```python
from build123d import *

# Parameters (mm, degrees)
SKETCH_1_R      = 16
SKETCH_1_R_2    = 4.5
SKETCH_1_R_3    = 1.85
EXTRUDE_1_DEPTH = 2


with BuildPart() as part:
    # 草图1 → 凸台-拉伸1 (new, symmetric)
    with BuildSketch(Plane.XY):
        Circle(SKETCH_1_R)
        Circle(SKETCH_1_R_2, mode=Mode.SUBTRACT)
        with Locations((-12, 0)):
            Circle(SKETCH_1_R_3, mode=Mode.SUBTRACT)
        with Locations((12, 0)):
            Circle(SKETCH_1_R_3, mode=Mode.SUBTRACT)
        with BuildLine():
            Line((-1, 6), (-1, 11))
            ThreePointArc((-1, 11), (0, 12), (1, 11))
            Line((1, 11), (1, 6))
            Line((1, 6), (-1, 6))
        make_face(mode=Mode.SUBTRACT)
        with BuildLine():
            Line((1, -6), (1, -11))
            ThreePointArc((1, -11), (0, -12), (-1, -11))
            Line((-1, -11), (-1, -6))
            Line((-1, -6), (1, -6))
        make_face(mode=Mode.SUBTRACT)
    extrude(amount=EXTRUDE_1_DEPTH, both=True)


solid = part.part
```
Read the model definition and answer for the solid it produces. Units are mm, in the model's axes. A direction names the side the tool comes from. Give positions to 0.01 mm unless a question says otherwise; leave off trailing zeros. Write each loop counter-clockwise with the first axis right and the second up, starting at its lowest first coordinate (ties: lowest second). Pieces come first, ordered by that corner, then holes. Notation, with made-up numbers: (-1, 12.5) -> (5, 12.5) arc R28 cw to (5, 45.5) -> close; hole circle Ø2 at (-7, -40). An arc over 180 degrees is marked (long way). Answer in a Markdown table with one row per item.
1) Section B-B on z = 0.8 is taken. Give the vertices of the cut face in (x, y).
Results list:
| item | result |
|---|---|
| outline | circle Ø32 at (0, 0); hole circle Ø3.7 at (-12, 0); hole circle Ø9 at (0, 0); hole (-1, -11) arc R1 ccw to (1, -11) -> (1, -6) -> (-1, -6) -> close; hole (-1, 6) -> (1, 6) -> (1, 11) arc R1 ccw to (-1, 11) -> close; hole circle Ø3.7 at (12, 0) |
2) Each of these flat-tipped pins is pushed along its axis until it touches: pin 1 Ø2 at (x, z) = (8, -1.5) entering from -Y; pin 2 Ø8 at (x, y) = (0, 0) entering from +Z. Where does it stop, or does it pass through?
Results list:
| item | result |
|---|---|
| pin 1 | y = -14.39 |
| pin 2 | through |
3) Section A-A on x = 0 is taken. Give the vertices of the cut face in (y, z).
Results list:
| item | result |
|---|---|
| outline | (-16, -2) -> (-12, -2) -> (-12, 2) -> (-16, 2) -> close; (-6, -2) -> (-4.5, -2) -> (-4.5, 2) -> (-6, 2) -> close; (4.5, -2) -> (6, -2) -> (6, 2) -> (4.5, 2) -> close; (12, -2) -> (16, -2) -> (16, 2) -> (12, 2) -> close |
4) Section C-C on y = 10 is taken. Give the vertices of the cut face in (x, z), plus the area to 3 significant figures.
Results list:
| item | result |
|---|---|
| outline | (-12.49, -2) -> (-1, -2) -> (-1, 2) -> (-12.49, 2) -> close; (1, -2) -> (12.49, -2) -> (12.49, 2) -> (1, 2) -> close |
| area | 91.9 mm^2 |
5) Section D-D on x = -4 is taken. Give the vertices of the cut face in (y, z).
Results list:
| item | result |
|---|---|
| outline | (-15.49, -2) -> (-2.06, -2) -> (-2.06, 2) -> (-15.49, 2) -> close; (2.06, -2) -> (15.49, -2) -> (15.49, 2) -> (2.06, 2) -> close |
6) A tool of negligible diameter and unlimited length cuts with its end or side. For faces 1 (the flat face through (3.3, -3.3, 2)), 2 (the flat face through (-1, -9, 0)), from which of +Z, -Z, +X, -X, +Y, -Y can it reach the whole face along a straight path? Write none if from no direction.
Results list:
| item | result |
|---|---|
| face 1 | +Z, +X, -X, +Y, -Y |
| face 2 | +Z, -Z |
7) Straight lines are drawn through the part: line 1 (X direction, y = -1, z = -0.65); line 2 (X direction, y = -1.5, z = 1.1); line 3 (Y direction, x = 13, z = -0.65). For each, find the intervals that lie inside material, in ascending order. Write a range as [from, to].
Results list:
| item | result |
|---|---|
| line 1 | [-15.97, -13.56], [-10.44, -4.39], [4.39, 10.44], [13.56, 15.97] |
| line 2 | [-15.93, -13.08], [-10.92, -4.24], [4.24, 10.92], [13.08, 15.93] |
| line 3 | [-9.33, -1.56], [1.56, 9.33] |
8) Determine the mould class of faces 3 (the flat face through (3.3, -3.3, -2)), 4 (the cylindrical face through (-3.47, -15.62, 0.03)), 5 (the flat face through (1, 9, 0)) for opening direction Y: released by +Y, released by -Y, zero draft, split by the parting line, or undercut.
Results list:
| item | result |
|---|---|
| face 3 | zero draft |
| face 4 | split by the parting line |
| face 5 | undercut |
